```python
from build123d import *

# Parameters (mm, degrees)
BOSS_EXTRU_1_DEPTH = 5.33
ESQUISSE2_W        = 0.51
ESQUISSE2_H        = 0.56
BOSS_EXTRU_2_DEPTH = 12.7


with BuildPart() as part:
    # Esquisse1 → Boss.-Extru.1 (new body)
    with BuildSketch(Plane.XY):
        with BuildLine():
            Line((-1.27, 2.105), (-1.27, -2.105))
            Line((-1.27, -2.105), (0, -2.585884762))
            ThreePointArc((0, -2.585884762), (2.92, 0), (0, 2.585884762))
            Line((0, 2.585884762), (-1.27, 2.105))
        make_face()
    extrude(amount=BOSS_EXTRU_1_DEPTH)

    # Esquisse2 → Boss.-Extru.2 (add)
    with BuildSketch(Plane(origin=(0, 0, 0), x_dir=(-1, 0, 0), z_dir=(0, 0, -1))):
        with Locations((0, 1.34)):
            Rectangle(ESQUISSE2_W, ESQUISSE2_H)
        Rectangle(ESQUISSE2_W, ESQUISSE2_H)
        with Locations((0, -1.34)):
            Rectangle(ESQUISSE2_W, ESQUISSE2_H)
    extrude(amount=BOSS_EXTRU_2_DEPTH)


solid = part.part
```
Geometry check sheet. Reference: the model listing, model coordinates, mm. Coordinates: 2 decimals unless noted, no trailing zeros. Loops run counter-clockwise (first coordinate to the right, second up) from the corner with the lowest first, then second, coordinate; pieces in that order, holes last.
Item 1: Go/stop test with flat-tipped pins: pin 1 Ø0.6 at (y, z) = (0, -7.5) entering from -X (3 decimals); pin 2 Ø1.5 at (x, z) = (1.5, -4.5) entering from -Y. Record where each tip stops, or that it passes through.
Item 2: Thickness scan on line 1 (Y direction, x = 0.2, z = -0.5); line 2 (X direction, y = -1.15, z = -2) (3 decimals); line 3 (Z direction, x = -0.55, y = 0.75). Record the ranges inside material, lowest first.
Item 3: Sectioned sample at D-D, the plane x = 0.45. Record the boundary of the cut face in (y, z), then the cut area to 3 significant figures.
Item 4: Sectioned sample at C-C, the plane z = 0.5. Record the boundary of the cut face in (x, y) (3 decimals), then the cut area to 3 significant figures.
Item 5: Sectioned sample at B-B, the plane y = 0. Record the boundary of the cut face in (x, z) (3 decimals).
Item 6: Sectioned sample at A-A, the plane z = -9.25. Record the boundary of the cut face in (x, y) (3 decimals), then the cut area to 3 significant figures.
Check result:
1. pin 1: stops at x = -0.255
1. pin 2: passes through
2. line 1: y = -1.62 to -1.06, -0.28 to 0.28, 1.06 to 1.62
2. line 2: x = -0.255 to 0.255
2. line 3: z = 0 to 5.33
3. outline: (-2.6, 0) - (2.6, 0) - (2.6, 5.33) - (-2.6, 5.33) - close
3. area: 27.7 mm2
4. outline: (-1.27, -2.105) - (0, -2.586) arc R2.605 ccw (long way) to (0, 2.586) - (-1.27, 2.105) - close
4. area: 18.3 mm2
5. outline: (-1.27, 0) - (-0.255, 0) - (-0.255, -12.7) - (0.255, -12.7) - (0.255, 0) - (2.92, 0) - (2.92, 5.33) - (-1.27, 5.33) - close
6. outline: (-0.255, -1.62) - (0.255, -1.62) - (0.255, -1.06) - (-0.255, -1.06) - close; (-0.255, -0.28) - (0.255, -0.28) - (0.255, 0.28) - (-0.255, 0.28) - close; (-0.255, 1.06) - (0.255, 1.06) - (0.255, 1.62) - (-0.255, 1.62) - close
6. area: 0.857 mm2
